Verification items for the finished model (mm, model axes). A direction names the side the tool comes from. Give positions to 0.01 mm unless a question says otherwise; leave off trailing zeros. Write each loop counter-clockwise with the first axis right and the second up, starting at its lowest first coordinate (ties: lowest second). Pieces come first, ordered by that corner, then holes. Notation, with made-up numbers: (-7, 53.5) - (1, 53.5) arc R12 ccw to (1, 66.5) - close; hole circle Ø4 at (81, -39). An arc over 180 degrees is marked (long way). Answer as a JSON object with one key per item and string values. Group by question number.
Item 1: Sectioned sample at D-D, the plane x = 10.5. Record the boundary of the cut face in (y, z) (1 decimal), and give its area (3 significant figures).
Item 2: Draft check along X on faces 4 (the face through (14.225, 8.748, 0.052)), 5 (the face through (-37.059, 1, 0)), 6 (the face through (-5.31, 8.75, -0.05)), 7 (the face through (33, 9, -2.381)). Enter one of: +X half, -X half, draft (parallel to the pull), parting line (faces both ways), or undercut.
Item 3: Scan lines: line 1 along Y through (x, z) = (54.5, 0); line 2 along X through (y, z) = (6, 5.75); line 3 along Z through (x, y) = (52.5, 1.5). Record each from-to range of solid material in increasing order. Write a range as [from, to].
Item 4: Sectioned sample at C-C, the plane z = -6.25. Record the boundary of the cut face in (x, y).
Item 5: Sectioned sample at A-A, the plane y = 4. Record the boundary of the cut face in (x, z).
Item 6: Go/stop test with flat-tipped pins: pin 1 (1.4 mm diameter, centred on x = -24.5, z = 1, fed in from +Y); pin 2 (1.2 mm diameter, centred on x = -24.5, y = 9.5, fed in from +Z); pin 3 (2.5 mm diameter, centred on x = 36, y = 8.5, fed in from +Z); pin 4 (2 mm diameter, centred on y = -6.5, z = 6, fed in from +X). Record where each tip stops, or that it passes through.
Item 7: Sectioned sample at B-B, the plane x = 46. Record the boundary of the cut face in (y, z) (1 decimal).
Item 8: Tool access check on faces 1 (the face through (34, 9, 2.381)), 2 (the face through (57.43, -2.44, -0.54)), 3 (the face through (-23, 9, -2.381)). Record the directions out of +Z, -Z, +X, -X, +Y, -Y that give a thin tool (end or side, any length) a straight path to the whole face; none if there is none.
```python
from build123d import *

# Parameters (mm, degrees)
SKETCH1_R             = 10.033
BOSS_EXTRUDE1_DEPTH   = 2.1336
SKETCH2_R             = 7.9375
BOSS_EXTRUDE2_DEPTH   = 65.024
M6_TAPPED_HOLE1_D     = 5
M6_TAPPED_HOLE1_DEPTH = 14.986
M6_TAPPED_HOLE1_TIP   = 1.502151548
BOSS_EXTRUDE3_START   = 34.925
SKETCH5_R             = 7.9375
BOSS_EXTRUDE3_DEPTH   = 34.925
BOSS_EXTRUDE4_DEPTH   = 4.7625


with BuildPart() as part:
    # Sketch1 → Boss-Extrude1 (new body)
    with BuildSketch(Plane(origin=(0, 0, 0), x_dir=(0, 0, -1), z_dir=(1, 0, 0))):
        Circle(SKETCH1_R)
    extrude(amount=-BOSS_EXTRUDE1_DEPTH)

    # Sketch2 → Boss-Extrude2 (add)
    with BuildSketch(Plane(origin=(0, 0, 0), x_dir=(0, 0, -1), z_dir=(1, 0, 0))):
        Circle(SKETCH2_R)
    extrude(amount=BOSS_EXTRUDE2_DEPTH)

    # M6 Tapped Hole1
    with Locations(Plane(origin=(65.024, 0, 0), x_dir=(0, 0, -1), z_dir=(1, 0, 0))):
        with Locations((0, 0)):
            Hole(M6_TAPPED_HOLE1_D / 2, depth=M6_TAPPED_HOLE1_DEPTH)
            with Locations((0, 0, -(M6_TAPPED_HOLE1_DEPTH + M6_TAPPED_HOLE1_TIP / 2))):  # 118° drill point
                Cone(0, M6_TAPPED_HOLE1_D / 2, M6_TAPPED_HOLE1_TIP, mode=Mode.SUBTRACT)

    # Sketch5 → Boss-Extrude3 (add)
    with BuildSketch(Plane.ZY.offset(2.1336).offset(BOSS_EXTRUDE3_START)):
        with Locations(Location((0, 0, 0), (0, 0, 180))):
            Circle(SKETCH5_R)
    extrude(amount=-BOSS_EXTRUDE3_DEPTH)

    # Sketch7 → Boss-Extrude4 (add)
    with BuildSketch(Plane(origin=(0, 5.1943, 0), x_dir=(1, 0, 0), z_dir=(0, 1, 0))):
        with BuildLine():
            Line((16.60525, 2.38125), (49.94275, 2.38125))
            ThreePointArc((49.94275, 2.38125), (52.324, 0), (49.94275, -2.38125))
            Line((49.94275, -2.38125), (16.60525, -2.38125))
            ThreePointArc((16.60525, -2.38125), (14.224, 0), (16.60525, 2.38125))
        make_face()
        with BuildLine():
            Line((-37.0586, 2.38125), (-7.68985, 2.38125))
            ThreePointArc((-7.68985, 2.38125), (-5.3086, 0), (-7.68985, -2.38125))
            Line((-7.68985, -2.38125), (-37.0586, -2.38125))
            Line((-37.0586, -2.38125), (-37.0586, 2.38125))
        make_face()
    extrude(amount=BOSS_EXTRUDE4_DEPTH)


solid = part.part
```
Geometry check:
{
 "1": {"outline": "circle Ø15.9 at (0, 0)", "area": "198 mm^2"},
 "2": {"face 4": "undercut", "face 5": "-X half", "face 6": "undercut", "face 7": "draft"},
 "3": {"line 1": "[-7.94, -2.5], [2.5, 7.94]", "line 2": "[-2.13, 0]", "line 3": "[-7.79, -2], [2, 7.79]"},
 "4": {"outline": "(-37.06, -4.89) - (-2.13, -4.89) - (-2.13, -7.85) - (0, -7.85) - (0, -4.89) - (65.02, -4.89) - (65.02, 4.89) - (0, 4.89) - (0, 7.85) - (-2.13, 7.85) - (-2.13, 4.89) - (-37.06, 4.89) - close"},
 "5": {"outline": "(-37.06, -6.86) - (-2.13, -6.86) - (-2.13, -9.2) - (0, -9.2) - (0, -6.86) - (65.02, -6.86) - (65.02, 6.86) - (0, 6.86) - (0, 9.2) - (-2.13, 9.2) - (-2.13, 6.86) - (-37.06, 6.86) - close"},
 "6": {"pin 1": "y = 9.96", "pin 2": "z = 2.38", "pin 3": "z = 3.23", "pin 4": "x = 65.02"},
 "7": {"outline": "(7.6, -2.4) - (10, -2.4) - (10, 2.4) - (7.6, 2.4) arc R7.9 ccw (long way) to start"},
 "8": {"face 1": "+Z, +X, +Y", "face 2": "+X", "face 3": "-Z, -X, +Y"}
}
